Design review of the part built by this model. Coordinates are the model's own, in mm. A direction names the side the tool comes from. Round coordinates to 2 decimals unless told otherwise and drop trailing zeros. Loops run counter-clockwise (first coordinate to the right, second up) from the corner with the lowest first, then second, coordinate; pieces in that order, holes last. Notation, with made-up numbers: (83.5, 42.25) -> (107.5, 42.25) arc R21 cw to (107.5, 73.25) -> close; hole circle Ø1 at (53.5, 57). An arc over 180 degrees is marked (long way). Write each question's results on one line, items separated by ' | '. Start each with the question number.
from build123d import *

# Parameters (mm, degrees)
SKETCH_1_W                   = 164
SKETCH_1_H                   = 225
SM_BASE_FLANGE_1_DEPTH       = 2
SM_START                     = -2
SM_EDGE_FLANGE_1_DEPTH       = 5
SM_START_2                   = -18
SM_EDGE_FLANGE_1_2_OUTLINE_W = 140
SM_EDGE_FLANGE_1_2_OUTLINE_H = 2
SM_EDGE_FLANGE_1_2_DEPTH     = 16
SM_START_3                   = -70
SM_EDGE_FLANGE_1_3_DEPTH     = 140
SM_EDGE_FLANGE_1_4_DEPTH     = 140
HOLE_WIZARD_M61_AT_2_COUNT   = 2
HOLE_WIZARD_M61_AT_2_PITCH   = 50
HOLE_WIZARD_M61_AT_3_COUNT   = 2
HOLE_WIZARD_M61_AT_3_PITCH   = 50
HOLE_WIZARD_M61_2_D          = 6.5
CUT_EXTRUDE_1_REACH          = 148.302
SKETCH_10_W                  = 88
SKETCH_10_H                  = 92
CHAMFER_1_SIZE               = 10


with BuildPart() as part:
    # Базовая кромка1: sheet metal written as solids
    # Sketch 1 → Базовая кромка1 (new body)
    with BuildSketch(Plane(origin=(0, 0, 0), x_dir=(1, 0, 0), z_dir=(0, 1, 0))):
        with Locations((0, 7)):
            Rectangle(SKETCH_1_W, SKETCH_1_H)
    extrude(amount=SM_BASE_FLANGE_1_DEPTH)

    # Ребро-кромка1: read off the stored shape, not the designer's step
    # Ребро-кромка1 outline → Ребро-кромка1 (cut)
    with BuildSketch(Plane(origin=(0, 0, 0), x_dir=(1, 0, 0), z_dir=(0, 1, 0)).offset(SM_START)):
        with BuildLine():
            Line((-70, 114.5), (-70, 119.5))
            Line((-70, 119.5), (-71, 119.5))
            Line((-71, 119.5), (-71, 114.5))
            ThreePointArc((-71, 114.5), (-70.5, 114), (-70, 114.5))
        make_face()
        with BuildLine():
            Line((71, 119.5), (70, 119.5))
            Line((70, 119.5), (70, 114.5))
            ThreePointArc((70, 114.5), (70.5, 114), (71, 114.5))
            Line((71, 114.5), (71, 119.5))
        make_face()
    extrude(amount=SM_EDGE_FLANGE_1_DEPTH, mode=Mode.SUBTRACT)

    # Sm Edge Flange 1 3 outline → Sm Edge Flange 1 3 (cut)
    with BuildSketch(Plane.YZ.offset(SM_START_3)):
        with BuildLine():
            ThreePointArc((2, -115.5), (1.464101615, -117.5), (0, -118.964101616))
            Line((0, -118.964101616), (0, -119.5))
            Line((0, -119.5), (2, -119.5))
            Line((2, -119.5), (2, -115.5))
        make_face()
    extrude(amount=SM_EDGE_FLANGE_1_3_DEPTH, mode=Mode.SUBTRACT)



with BuildPart() as body_2:
    # Sm Edge Flange 1 2 outline → Sm Edge Flange 1 2 (new body)
    with BuildSketch(Plane(origin=(0, 0, 0), x_dir=(1, 0, 0), z_dir=(0, 1, 0)).offset(SM_START_2)):
        with Locations((0, 118.5)):
            Rectangle(SM_EDGE_FLANGE_1_2_OUTLINE_W, SM_EDGE_FLANGE_1_2_OUTLINE_H)
    extrude(amount=SM_EDGE_FLANGE_1_2_DEPTH)


with BuildPart() as part_1:
    add(part.part)

    add(body_2.part)  # Sm Edge Flange 1 4 merges body 2
    # Sm Edge Flange 1 4 outline → Sm Edge Flange 1 4 (add)
    with BuildSketch(Plane.YZ.offset(SM_START_3)):
        with BuildLine():
            Line((-2, -117.5), (-2, -119.5))
            ThreePointArc((-2, -119.5), (-0.96472382, -119.363703305), (0, -118.964101616))
            Line((0, -118.964101616), (0, -115.5))
            ThreePointArc((0, -115.5), (-0.585786438, -116.914213562), (-2, -117.5))
        make_face()
    extrude(amount=SM_EDGE_FLANGE_1_4_DEPTH)

    # Эскиз7 → Hole Wizard M61 (revolve, cut)
    with BuildSketch(Plane(origin=(0, -10, -119.5), x_dir=(0, 1, 0), z_dir=(1, 0, 0))):
        Polygon((0, 0), (0, 2), (4.5, 2), (4.5, 1.5), (6, 0), align=None)
    hole_wizard_m61 = revolve(axis=Axis((0, -10, -125.85), (0, 0, 1)), mode=Mode.SUBTRACT)

    # Hole Wizard M61 at 2: Hole Wizard M61 ×2
    with Locations(*[(i * HOLE_WIZARD_M61_AT_2_PITCH, 0, 0) for i in range(1, HOLE_WIZARD_M61_AT_2_COUNT)]):
        add(hole_wizard_m61, mode=Mode.SUBTRACT)

    # Hole Wizard M61 at 3: Hole Wizard M61 ×2
    with Locations(*[(-i * HOLE_WIZARD_M61_AT_3_PITCH, 0, 0) for i in range(1, HOLE_WIZARD_M61_AT_3_COUNT)]):
        add(hole_wizard_m61, mode=Mode.SUBTRACT)

    # Hole Wizard M61 2 (through all)
    with Locations(Plane(origin=(-76, 2, 44.5), x_dir=(0, 0, 1), z_dir=(0, 1, 0))):
        with Locations((0, 0), (-110, 0), (-110, 152), (0, 152), (17, 126), (17, 26), (55, 34), (55, 118), (55, 76), (17, 76), (-55, 152), (-55, 0)):
            Hole(HOLE_WIZARD_M61_2_D / 2)

    # Эскиз10 → Вытянуть1 (cut, up to next)
    with BuildSketch(Plane(origin=(0, 2, 0), x_dir=(1, 0, 0), z_dir=(0, 1, 0)), mode=Mode.PRIVATE) as cut_extrude_1_sk1:
        Rectangle(SKETCH_10_W, SKETCH_10_H)
    cut_extrude_1_tool1 = extrude(cut_extrude_1_sk1.sketch, amount=-CUT_EXTRUDE_1_REACH, mode=Mode.PRIVATE) & part_1.part
    add(cut_extrude_1_tool1.solids().sort_by_distance((0, 2, 0))[0], mode=Mode.SUBTRACT)

    # Фаска1
    chamfer_1_edges = [part_1.edges().sort_by_distance(p)[0] for p in [
        (-82, 1, -119.5),
        (82, 1, -119.5),
        (82, 1, 105.5),
        (-82, 1, 105.5),
    ]]
    chamfer(chamfer_1_edges, length=CHAMFER_1_SIZE)


solid = part_1.part
1) Take a section at D-D (x = 27.5). Write out the cut boundary in (y, z).
2) Insertion check: pin 1 (6 mm diameter, centred on x = -50, y = -5, fed in from -Z); pin 2 (11.5 mm diameter, centred on x = -50, y = -10, fed in from -Z); pin 3 (1 mm diameter, centred on x = -11.5, y = 0.5, fed in from -Z); pin 4 (8.5 mm diameter, centred on x = -50, z = 61.5, fed in from -Y). Each pin has a flat end and moves straight along its axis. Give the tip position at first contact, or say it passes through.
3) Take a section at C-C (z = 35.5). Write out the cut boundary in (x, y), plus the area to 3 significant figures.
4) Take a section at B-B (x = -50). Write out the cut boundary in (y, z).
5) The part is to be moulded in two halves that separate along Y. For faces 4 (the face through (-1, 2, -59)), 5 (the face through (54.39, -10.98, -117.75)), 6 (the face through (74.022, 0.986, -7.921)), say which applies: +Y half, -Y half, draft (parallel to the pull), parting line (faces both ways), or undercut.
6) Take a section at A-A (z = 99.5). Write out the cut boundary in (x, y), plus the area to 3 significant figures.
7) For faces 1 (the face through (-77.245, 0.986, 41.498)), 2 (the face through (70, -8, -118)), 3 (the face through (-1, 0, -59)), list the 3-axis set-ups (+Z, -Z, +X, -X, +Y, -Y) from which the entire face can be reached by the end or side of a thin tool; tool diameter is ignored.
8) To check wall thickness, follow line 1 (X direction, y = 1.05, z = 44.5); line 2 (X direction, y = -10, z = -117.6); line 3 (Y direction, x = 18.5, z = -102.5). State the ranges of each line that lie inside material, in increasing order. Write a range as from..to.
Geometry check:
1) outline: (-18, -119.5) -> (-2, -119.5) arc R4 ccw to (2, -115.5) -> (2, -46) -> (0, -46) -> (0, -115.5) arc R2 cw to (-2, -117.5) -> (-18, -117.5) -> close; (0, 46) -> (2, 46) -> (2, 105.5) -> (0, 105.5) -> close
2) pin 1: stops at z = -119.5 | pin 2: stops at z = -119.25 | pin 3: stops at z = -118.96 | pin 4: stops at y = 0
3) outline: (-82, 0) -> (-44, 0) -> (-44, 2) -> (-82, 2) -> close; (44, 0) -> (82, 0) -> (82, 2) -> (44, 2) -> close | area: 152 mm^2
4) outline: (-18, -119.5) -> (-16, -119.5) -> (-14.5, -118) -> (-14.5, -117.5) -> (-18, -117.5) -> close; (-5.5, -118) -> (-4, -119.5) -> (-2, -119.5) arc R4 ccw to (2, -115.5) -> (2, 58.25) -> (0, 58.25) -> (0, -115.5) arc R2 cw to (-2, -117.5) -> (-5.5, -117.5) -> close; (0, 64.75) -> (2, 64.75) -> (2, 105.5) -> (0, 105.5) -> close
5) face 4: +Y half | face 5: undercut | face 6: draft
6) outline: (-78, 0) -> (-45.25, 0) -> (-45.25, 2) -> (-78, 2) -> close; (-38.75, 0) -> (-3.25, 0) -> (-3.25, 2) -> (-38.75, 2) -> close; (3.25, 0) -> (38.75, 0) -> (38.75, 2) -> (3.25, 2) -> close; (45.25, 0) -> (78, 0) -> (78, 2) -> (45.25, 2) -> close | area: 273 mm^2
7) face 1: +Y, -Y | face 2: -Z, +Y, -Y | face 3: +Z, +X, -X, -Y
8) line 1: x = -82..-79.25, -72.75..-44, 44..72.75, 79.25..82 | line 2: x = -70..-54.5, -45.5..-4.5, 4.5..45.5, 54.5..70 | line 3: y = 0..2
